Input: dimensioned drawing with shaded views. Units: mm. Origin: part minimum x, y, z. A direction names the side the tool comes from. Give positions to 0.01 mm unless a question says otherwise; leave off trailing zeros. Write each loop counter-clockwise with the first axis right and the second up, starting at its lowest first coordinate (ties: lowest second). Pieces come first, ordered by that corner, then holes. Notation, with made-up numbers: (11.5, 38) - (45.5, 38) arc R24 cw to (45.5, 77) - close; hole circle Ø11 at (11.5, -13). An arc over 180 degrees is marked (long way). Answer as CSV lines item,"result".
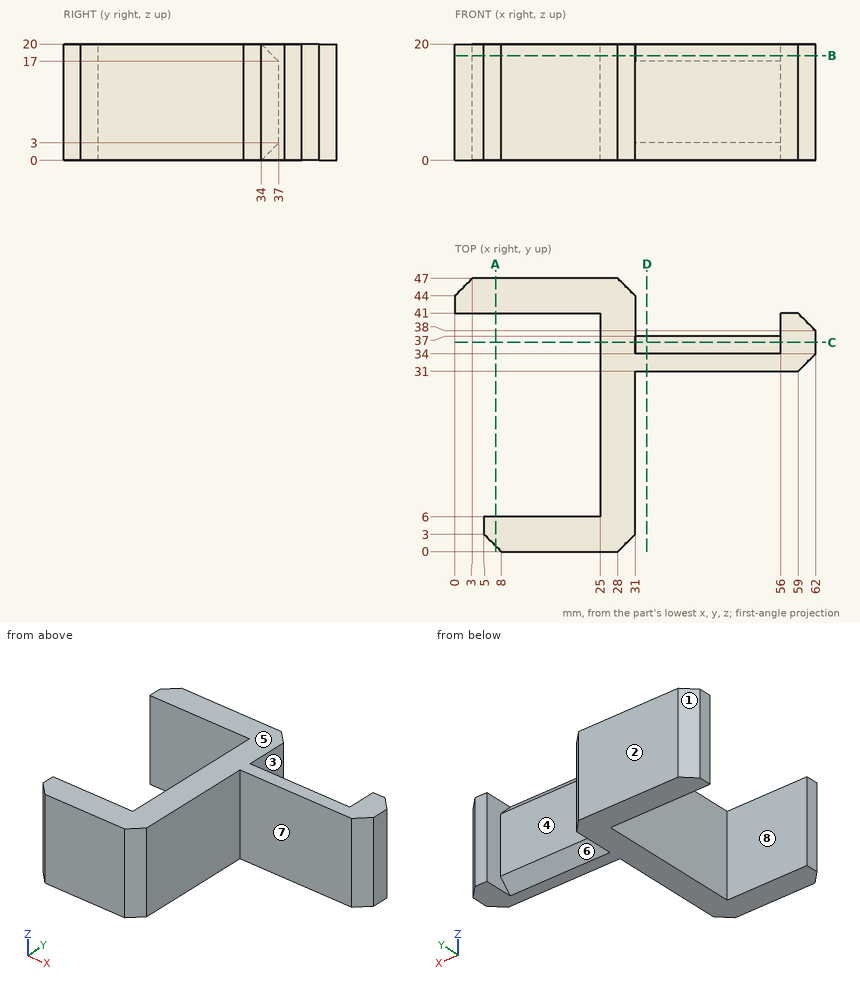
Item 1: Cut plane B-B on z = 18. Return the cut outline in (x, y), plus the area to 3 significant figures.
The answers:
outline,"(0, 41) - (25, 41) - (25, 6) - (5, 6) - (5, 3) - (8, 0) - (28, 0) - (31, 3) - (31, 31) - (59, 31) - (62, 34) - (62, 38) - (59, 41) - (56, 41) - (56, 36) - (31, 36) - (31, 44) - (28, 47) - (3, 47) - (0, 44) - close"
area,"710 mm²"
Item 2: Cut plane D-D on x = 33. Return the cut outline in (y, z), plus the area to 3 significant figures.
The answers:
outline,"(31, 0) - (34, 0) - (37, 3) - (37, 17) - (34, 20) - (31, 20) - close"
area,"111 mm²"
Item 3: Reachability of the marked faces 4, 5, 6, 7 and 8 from +Z, -Z, +X, -X, +Y, -Y: full face, straight path, thin tool, end or side. Return the list, or none.
The answers:
face 4,"+Z, -Z, +Y"
face 5,"+Z, +X, -X, +Y, -Y"
face 6,"-Z, +Y"
face 7,"+Z, -Z, +X, -Y"
face 8,"+Z, -Z, -X"
Item 4: Cut plane A-A on x = 7. Return the cut outline in (y, z).
The answers:
outline,"(1, 0) - (6, 0) - (6, 20) - (1, 20) - close; (41, 0) - (47, 0) - (47, 20) - (41, 20) - close"
Item 5: Cut plane C-C on y = 36. Return the cut outline in (x, z).
The answers:
outline,"(25, 0) - (31, 0) - (31, 2) - (56, 2) - (56, 0) - (62, 0) - (62, 20) - (56, 20) - (56, 18) - (31, 18) - (31, 20) - (25, 20) - close"
Item 6: Contact query for flat-ended pins moving along their axis: pin 1 (3.5 mm diameter, centred on x = 58, z = 7, fed in from +Y); pin 2 (8 mm diameter, centred on y = 6.5, z = 4.5, fed in from +X); pin 3 (5.5 mm diameter, centred on y = 37, z = 12.5, fed in from -X). Output: stop coordinate, or through.
The answers:
pin 1,"y = 41"
pin 2,"x = 31"
pin 3,"x = 25"
Item 7: Mould query, pull axis X, two halves, no side actions, for the marked faces 1, 2 and 3. Classes: +X half, -X half, draft (parallel to the pull), parting line (faces both ways), or undercut.
The answers:
face 1,"-X half"
face 2,"draft"
face 3,"undercut"
Item 8: Ray query, line 1 (X direction, y = 37, z = 1.5); line 2 (Y direction, x = 23, z = 18.25); line 3 (X direction, y = 3, z = 17.25). Return the intervals inside material, ascending. Write a range as from..to.
The answers:
line 1,"25..31, 56..62"
line 2,"0..6, 41..47"
line 3,"5..31"
